Work out the finished part from the listing and answer in its coordinate system (mm). A direction names the side the tool comes from. Round coordinates to 2 decimals unless told otherwise and drop trailing zeros. Loops run counter-clockwise (first coordinate to the right, second up) from the corner with the lowest first, then second, coordinate; pieces in that order, holes last. Notation, with made-up numbers: M 85,49 L 128,49 A22 cw 128,84 Z; hole C 1,88 d4. An arc over 180 degrees is marked long. One line per item, written item: value.
```python
from build123d import *

# Parameters (mm, degrees)
SKETCH1_W               = 20
SKETCH1_H               = 30
BOSS_EXTRUDE1_DEPTH     = 40
SKETCH2_R               = 4.25
CUT_EXTRUDE1_DEPTH      = 15
CUT_EXTRUDE2_DEPTH      = 44.874821937
CUT_EXTRUDE2_DEPTH_BACK = 44.874821937
SKETCH11_R              = 5
FILLET1_R               = 10


with BuildPart() as part:
    # Sketch1 → Boss-Extrude1 (new body)
    with BuildSketch(Plane(origin=(0, 0, 0), x_dir=(1, 0, 0), z_dir=(0, 1, 0))):
        Rectangle(SKETCH1_W, SKETCH1_H)
    extrude(amount=-BOSS_EXTRUDE1_DEPTH)

    # Sketch2 → Cut-Extrude1 (cut)
    with BuildSketch(Plane(origin=(0, 0, 0), x_dir=(1, 0, 0), z_dir=(0, 1, 0))):
        with Locations(Location((0, 0, 0), (0, 0, 270))):
            Circle(SKETCH2_R)
    extrude(amount=-CUT_EXTRUDE1_DEPTH, mode=Mode.SUBTRACT)

    # Sketch11 → Cut-Extrude2 (cut, two sides: drawn at the far end of the back side and taken through both)
    with BuildSketch(Plane(origin=(0, 0, 0), x_dir=(0, 0, -1), z_dir=(1, 0, 0)).offset(-CUT_EXTRUDE2_DEPTH_BACK)):
        with Locations((0, -25)):
            Circle(SKETCH11_R)
    extrude(amount=CUT_EXTRUDE2_DEPTH + CUT_EXTRUDE2_DEPTH_BACK, mode=Mode.SUBTRACT)

    # Fillet1
    fillet1_edges = [part.edges().sort_by_distance(p)[0] for p in [
        (0, -40, 15),
        (0, -40, -15),
    ]]
    fillet(fillet1_edges, radius=FILLET1_R)


solid = part.part
```
1) Find section C-C (z = 0). Give the vertices of the cut face in (x, y), then the cut area to 4 significant figures.
Check values:
outline: M -10,-40 L 10,-40 L 10,-30 L -10,-30 Z; M -10,-20 L 10,-20 L 10,0 L 4.25,0 L 4.25,-15 L -4.25,-15 L -4.25,0 L -10,0 Z
area: 472.5 mm2
2) For faces 1 (the face through (4.214, -7.395, -0.553)), 2 (the face through (10, -19.7, 0.2)), determine the directions among +Z, -Z, +X, -X, +Y, -Y from which every point of the face is accessible in a straight line to the end or side of a thin tool.
Check values:
face 1: +Y
face 2: +Z, -Z, +X, +Y, -Y
3) This flat-tipped pin is pushed along its axis until it touches: pin 1 (7 mm diameter, centred on x = 0, z = 0, fed in from +Y). Where does it stop, or does it pass through?
Check values:
pin 1: y = -15
4) Find section B-B (x = 0). Give the vertices of the cut face in (y, z).
Check values:
outline: M -40,-5 A10 ccw -30,-15 L 0,-15 L 0,-4.25 L -15,-4.25 L -15,4.25 L 0,4.25 L 0,15 L -30,15 A10 ccw -40,5 Z; hole C -25,0 d10
5) Find the intervals of material crossed by probe 1 along Y at (x, z) = (-1.25, 0); probe 2 along Y at (x, z) = (-5.5, 0); probe 3 along X at (y, z) = (-8, 0), in increasing order. Write a range as from..to.
Check values:
probe 1: -40..-30, -20..-15
probe 2: -40..-30, -20..0
probe 3: -10..-4.25, 4.25..10
6) The mould has two halves that part along Z. Classify faces 3 (the face through (0, -15, 0)), 4 (the face through (0, -15, 15)), 5 (the face through (0.14, -37.15, -11.99)): +Z half, -Z half, draft (parallel to the pull), parting line (faces both ways), or undercut.
Check values:
face 3: undercut
face 4: +Z half
face 5: -Z half
7) Find section A-A (y = -29). Give the vertices of the cut face in (x, z).
Check values:
outline: M -10,-15 L 10,-15 L 10,-3 L -10,-3 Z; M -10,3 L 10,3 L 10,15 L -10,15 Z
8) Find section D-D (y = -9.5). Give the vertices of the cut face in (x, z).
Check values:
outline: M -10,-15 L 10,-15 L 10,15 L -10,15 Z; hole C 0,0 d8.5
